from build123d import *

# Parameters (mm, degrees)
F1_DEPTH = 63.5
F2_DEPTH = 25.4
F3_DEPTH = 7.9375
F0_W     = 25.4
F0_H     = 19.05
F4_DEPTH = 25.4
F6_R     = 6.35


with BuildPart() as f1:
    # F0 (on Front) → F1 (new body, symmetric)
    with BuildSketch(Plane.XZ):
        with BuildLine():
            Line((-41.275, 9.2450247044), (-41.275, -9.525))
            Line((-41.275, -9.525), (41.275, -9.525))
            Line((41.275, -9.525), (41.275, 9.525))
            Line((41.275, 9.525), (22.225, 9.525))
            Line((22.225, 9.525), (-41.1268438883, 9.525))
            add(Edge.make_bspline(
                [(-41.275, 9.2450247044), (-41.2721793897, 9.2493286898), (-41.2526024622, 9.2855029924), (-41.1980769813, 9.3907074254), (-41.1268438883, 9.525)],
                knots=[0.0426221028, 0.0426221028, 0.0426221028, 0.0426221028, 0.0482250452, 0.0779432741, 0.0779432741, 0.0779432741, 0.0779432741], degree=3))
        make_face()
    extrude(amount=F1_DEPTH, both=True)

    # F0 (on Front) → F2 (join, symmetric)
    with BuildSketch(Plane.XZ):
        with BuildLine():
            Line((22.225, 9.525), (41.275, 9.525))
            Line((41.275, 9.525), (41.275, 27.0002))
            ThreePointArc((41.275, 27.0002), (45.9246798487, 38.2255201513), (57.15, 42.8752))
            Line((57.15, 42.8752), (60.325, 42.8752))
            Line((60.325, 42.8752), (60.325, 61.9252))
            Line((60.325, 61.9252), (57.15, 61.9252))
            ThreePointArc((57.15, 61.9252), (32.4542956671, 51.6959043329), (22.225, 27.0002))
            Line((22.225, 27.0002), (22.225, 9.525))
        make_face()
    extrude(amount=F2_DEPTH, both=True)

    # F0 (on Front) → F3 (join, symmetric)
    with BuildSketch(Plane.XZ):
        with BuildLine():
            add(Edge.make_bspline(
                [(-41.1268438883, 9.525), (-38.9167205077, 13.6916470796), (-12.2967160163, 61.9252), (57.15, 61.9252)],
                knots=[0.0779432741, 0.0779432741, 0.0779432741, 0.0779432741, 1, 1, 1, 1], degree=3))
            Line((-41.1268438883, 9.525), (22.225, 9.525))
            Line((22.225, 9.525), (22.225, 27.0002))
            ThreePointArc((22.225, 27.0002), (32.4542956671, 51.6959043329), (57.15, 61.9252))
        make_face()
    extrude(amount=F3_DEPTH, both=True)

    # F0 (on Front) → F4 (join, symmetric)
    with BuildSketch(Plane.XZ):
        with Locations((73.025, 52.4002)):
            Rectangle(F0_W, F0_H)
    extrude(amount=F4_DEPTH, both=True)

    # F0 (on Front) → F5 (revolve)
    with BuildSketch(Plane.XZ):
        Polygon((85.725, 66.675), (85.725, 61.9252), (85.725, 42.8752), (85.725, 38.1), (111.125, 38.1), (111.125, 66.675), align=None)
    revolve(axis=Axis((85.725, 0, 52.3875), (0, 0, 1)))

    # F6
    f6_edges = [f1.edges().sort_by_distance(p)[0] for p in [
        (41.275, -63.5, 0),
        (-41.275, -63.5, -0.139988),
        (-41.275, 63.5, -0.139988),
        (41.275, 63.5, 0),
    ]]
    fillet(f6_edges, radius=F6_R)


solid = f1.part
Geometry check sheet. Reference: the model listing, model coordinates, mm. A direction names the side the tool comes from. Coordinates: 2 decimals unless noted, no trailing zeros. Use a Markdown table: item, result. Add a question column.
1. Material ranges on L1, parallel to Z at x = -21, y = 46 (3 decimals); L2, parallel to X at y = 17.5, z = 24.5 (3 decimals); L3, parallel to X at y = -56, z = -5.5 (3 decimals), recorded low to high.
2. Go/stop test with flat-tipped pins: pin 1 Ø8.5 at (y, z) = (-18.5, 19.5) entering from -X (3 decimals); pin 2 Ø15 at (x, y) = (86.5, -12.5) entering from -Z; pin 3 Ø1 at (x, y) = (-16, -36.5) entering from +Z (3 decimals). Record where each tip stops, or that it passes through.
3. Mould release check, pull along X, two halves, no side actions. Record for faces 1 (the face through (-41.275, -1, 0)), 2 (the face through (41.275, -1, 4)), 3 (the face through (85, 0, 66.675)), 4 (the face through (60, 2, 42.875)): pulls with the +X half, pulls with the -X half, needs draft (parallel to the pull), parting line crosses it, or undercut.
4. Set-up check for faces 5 (the face through (46, -25.4, 42)), 6 (the face through (22.225, -17, 18)), 7 (the face through (60, 2, 61.925)): record each of +Z, -Z, +X, -X, +Y, -Y from which the full face is reachable in a straight line by a thin tool's end or side.
Filled sheet:
| question | item | result |
|---|---|---|
| 1 | L1 | -9.525 to 9.525 |
| 1 | L2 | 22.225 to 41.275 |
| 1 | L3 | -41.275 to 41.275 |
| 2 | pin 1 | x = 22.225 |
| 2 | pin 2 | z = 38.1 |
| 2 | pin 3 | z = 9.525 |
| 3 | face 1 | pulls with the -X half |
| 3 | face 2 | pulls with the +X half |
| 3 | face 3 | needs draft |
| 3 | face 4 | undercut |
| 4 | face 5 | +Z, +X, -X, -Y |
| 4 | face 6 | +Z, -X, -Y |
| 4 | face 7 | +Z, -X |
